Check sheet for the modelled part. Datum: model origin and axes. Units: mm. Face numbers are marked on the shaded views. A direction names the side the tool comes from. Give positions to 0.01 mm unless a question says otherwise; leave off trailing zeros. Write each loop counter-clockwise with the first axis right and the second up, starting at its lowest first coordinate (ties: lowest second). Pieces come first, ordered by that corner, then holes. Notation, with made-up numbers: M 60,87.5 L 116,87.5 A32 cw 116,119.5 Z; hole C 58.25,47.25 d4. An arc over 180 degrees is marked long. Write item = value, one per line. Start each with the question number.
1) Sectioned sample at D-D, the plane z = 1.15. Record the cut outline in (x, y), then the cut area to 3 significant figures.
2) Gauge pin test, flat ends, axial feed: pin 1 (1.5 mm diameter, centred on y = 9.5, z = 3.5, fed in from -X); pin 2 (2 mm diameter, centred on x = 13.5, z = 3.5, fed in from +Y); pin 3 (1.1 mm diameter, centred on x = 12.5, z = 3.5, fed in from +Y). Record the tip position at first contact, or that the pin passes through.
3) Draft check along X on the marked faces 1, 2 and 3. Enter one of: pulls with the +X half, pulls with the -X half, needs draft (parallel to the pull), parting line crosses it, or undercut.
4) Sectioned sample at B-B, the plane x = 10.75. Record the cut outline in (y, z).
5) Sectioned sample at A-A, the plane z = 3.25. Record the cut outline in (x, y), then the cut area to 3 significant figures.
6) Sectioned sample at C-C, the plane y = 6.75. Record the cut outline in (x, z), then the cut area to 3 significant figures.
7) Set-up check for the marked faces 4, 5 and 6: record each of +Z, -Z, +X, -X, +Y, -Y from which the full face is reachable in a straight line by a thin tool's end or side.
8) Scan lines: L1, parallel to X at y = 9, z = 1.45; L2, parallel to Y at x = 6.75, z = 3.85; L3, parallel to Y at x = 5.5, z = 0.55. Record each from-to range of solid material in increasing order.
from build123d import *

# Parameters (mm, degrees)
F0_W     = 21.1
F0_H     = 19.6
F1_DEPTH = 4
F2_W     = 21.1
F2_H     = 19.6
F2_W_2   = 18.3
F2_H_2   = 16.8
F3_DEPTH = 1.4
F4_W     = 15.1
F4_H     = 13.6
F5_DEPTH = 25
F6_R     = 2
F7_R     = 0.6
F8_R     = 1.4


with BuildPart() as f1:
    # F0 (on Top) → F1 (new body)
    with BuildSketch(Plane.XY):
        with Locations((10.55, 9.8)):
            Rectangle(F0_W, F0_H)
    extrude(amount=F1_DEPTH)

    # F2 (on face) → F3 (cut)
    with BuildSketch(Plane.XY.offset(4)):
        with Locations((10.55, 9.8)):
            Rectangle(F2_W, F2_H)
        with Locations((10.55, 9.8)):
            Rectangle(F2_W_2, F2_H_2, mode=Mode.SUBTRACT)
    extrude(amount=-F3_DEPTH, mode=Mode.SUBTRACT)

    # F4 (on face) → F5 (cut)
    with BuildSketch(Plane.XY.offset(4)):
        with Locations((10.55, 9.8)):
            Rectangle(F4_W, F4_H)
    extrude(amount=-F5_DEPTH, mode=Mode.SUBTRACT)

    # F6
    f6_edges = [f1.edges().sort_by_distance(p)[0] for p in [
        (21.1, 19.6, 1.3),
        (21.1, 0, 1.3),
        (0, 0, 1.3),
        (0, 19.6, 1.3),
    ]]
    fillet(f6_edges, radius=F6_R)

    # F7
    f7_edges = [f1.edges().sort_by_distance(p)[0] for p in [
        (3, 16.6, 2),
        (18.1, 16.6, 2),
        (18.1, 3, 2),
        (3, 3, 2),
    ]]
    fillet(f7_edges, radius=F7_R)

    # F8
    f8_edges = [f1.edges().sort_by_distance(p)[0] for p in [
        (1.4, 1.4, 3.3),
        (19.7, 1.4, 3.3),
        (19.7, 18.2, 3.3),
        (1.4, 18.2, 3.3),
    ]]
    fillet(f8_edges, radius=F8_R)


solid = f1.part
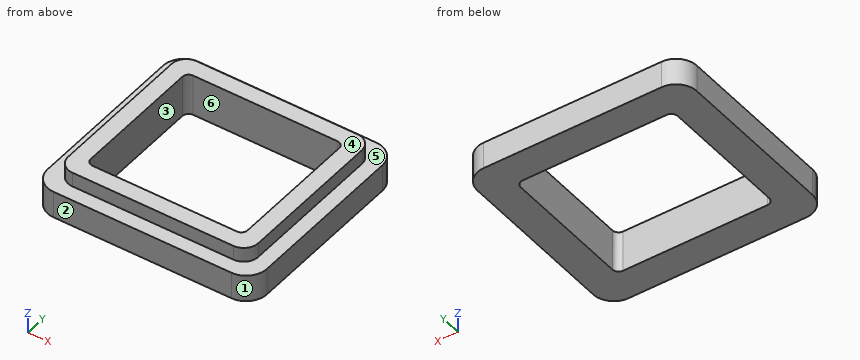
Data:
q1.outline = M 0,2 A2 ccw 2,0 L 19.1,0 A2 ccw 21.1,2 L 21.1,17.6 A2 ccw 19.1,19.6 L 2,19.6 A2 ccw 0,17.6 Z; hole M 3,3.6 A0.6 ccw 3.6,3 L 17.5,3 A0.6 ccw 18.1,3.6 L 18.1,16 A0.6 ccw 17.5,16.6 L 3.6,16.6 A0.6 ccw 3,16 Z
q1.area = 205 mm2
q2.pin_1 = 1.4
q2.pin_2 = 19.6
q2.pin_3 = 18.2
q3.face_1 = pulls with the +X half
q3.face_2 = needs draft
q3.face_3 = undercut
q4.outline = M 0,0 L 3,0 L 3,4 L 1.4,4 L 1.4,2.6 L 0,2.6 Z; M 16.6,0 L 19.6,0 L 19.6,2.6 L 18.2,2.6 L 18.2,4 L 16.6,4 Z
q5.outline = M 1.4,2.8 A1.4 ccw 2.8,1.4 L 18.3,1.4 A1.4 ccw 19.7,2.8 L 19.7,16.8 A1.4 ccw 18.3,18.2 L 2.8,18.2 A1.4 ccw 1.4,16.8 Z; hole M 3,3.6 A0.6 ccw 3.6,3 L 17.5,3 A0.6 ccw 18.1,3.6 L 18.1,16 A0.6 ccw 17.5,16.6 L 3.6,16.6 A0.6 ccw 3,16 Z
q5.area = 101 mm2
q6.outline = M 0,0 L 3,0 L 3,4 L 1.4,4 L 1.4,2.6 L 0,2.6 Z; M 18.1,0 L 21.1,0 L 21.1,2.6 L 19.7,2.6 L 19.7,4 L 18.1,4 Z
q6.area = 20.1 mm2
q7.face_4 = +Z, +X, -X, +Y, -Y
q7.face_5 = +Z
q7.face_6 = +Z, -Z
q8.L1 = 0 to 3, 18.1 to 21.1
q8.L2 = 1.4 to 3, 16.6 to 18.2
q8.L3 = 0 to 3, 16.6 to 19.6
